Could you check a few things on this model? Use its own coordinates, in mm. Face numbers are marked on the shaded views. A direction names the side the tool comes from. Coordinates: 2 decimals unless noted, no trailing zeros. Order: outer loops, then holes, each group sorted by start corner. A loop starts at its lowest first (then second) coordinate and runs counter-clockwise, first axis right, second up. Notation, with made-up numbers: (54, 27.5) - (78, 27.5) arc R22 ccw to (78, 51.5) - close; hole circle Ø6 at (29, 88). An arc over 180 degrees is marked (long way). One line per item, written item: value. Start each with the question number.
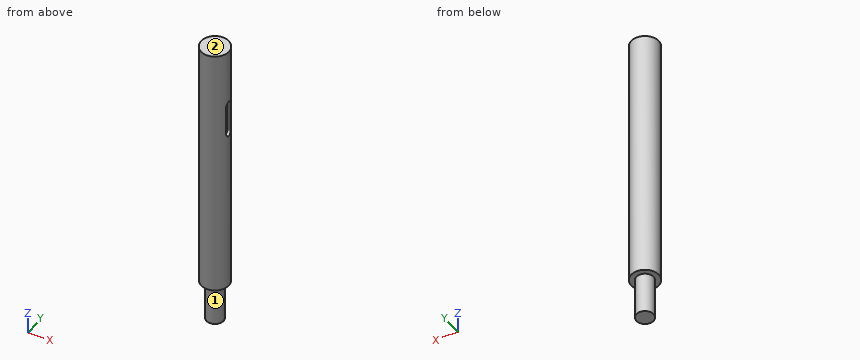
from build123d import *

# Parameters (mm, degrees)
SKETCH_1_R          = 4
EXTRUDE_1_DEPTH     = 75
SKETCH_2_R          = 2.5
EXTRUDE_2_DEPTH     = 12
CUT_EXTRUDE_1_DEPTH = 2


with BuildPart() as part:
    # ｽｹｯﾁ1 → ﾎﾞｽ - 押し出し1 (new body)
    with BuildSketch(Plane.XY):
        Circle(SKETCH_1_R)
    extrude(amount=EXTRUDE_1_DEPTH)

    # ｽｹｯﾁ2 → ﾎﾞｽ - 押し出し2 (add)
    with BuildSketch(Plane(origin=(0, 0, 0), x_dir=(-1, 0, 0), z_dir=(0, 0, -1))):
        Circle(SKETCH_2_R)
    extrude(amount=EXTRUDE_2_DEPTH)

    # ｽｹｯﾁ3 → ｶｯﾄ - 押し出し1 (cut, through all)
    with BuildSketch(Plane(origin=(3, 0, 0), x_dir=(0, 0, -1), z_dir=(1, 0, 0))):
        with BuildLine():
            Line((-57.9, 1.1), (-49.1, 1.1))
            ThreePointArc((-49.1, 1.1), (-48, 0), (-49.1, -1.1))
            Line((-49.1, -1.1), (-57.9, -1.1))
            ThreePointArc((-57.9, -1.1), (-59, 0), (-57.9, 1.1))
        make_face()
    extrude(amount=CUT_EXTRUDE_1_DEPTH, mode=Mode.SUBTRACT)


solid = part.part
Q1. I want a section at B-B on y = 0. Please give me the cut outline in (x, z), then the cut area to 3 significant figures.
Q2. I want a section at A-A on x = 0. Please give me the cut outline in (y, z).
Q3. I'm going to push flat-ended pins straight in: pin 1 (0.9 mm diameter, centred on x = 3, z = 52, fed in from -Y); pin 2 (1.1 mm diameter, centred on y = 0, z = 56, fed in from +X); pin 3 (2 mm diameter, centred on y = 2.5, z = 58.5, fed in from +X). Where does each tip first touch, or does it pass through?
Q4. Which directions (+Z, -Z, +X, -X, +Y, -Y) give clear straight access to the entire face, cutting with the end or side of a thin tool? Please do the marked faces 1 and 2.
Q5. I want a section at C-C on z = 31. Please give me the cut outline in (x, y).
Q6. If I drill on L1, parallel to Z at x = 0, y = 3; L2, parallel to Z at x = 3.5, y = -0.5; L3, parallel to Y at x = 3.5, z = 52, over which ranges is the centre line in solid material (lowest first)?
Values follow:
1. outline: (-4, 0) - (-2.5, 0) - (-2.5, -12) - (2.5, -12) - (2.5, 0) - (4, 0) - (4, 48) - (3, 48) - (3, 59) - (4, 59) - (4, 75) - (-4, 75) - close
1. area: 649 mm^2
2. outline: (-4, 0) - (-2.5, 0) - (-2.5, -12) - (2.5, -12) - (2.5, 0) - (4, 0) - (4, 75) - (-4, 75) - close
3. pin 1: stops at y = -3.08
3. pin 2: stops at x = 3
3. pin 3: stops at x = 3.71
4. face 1: -Z
4. face 2: +Z, +X, -X, +Y, -Y
5. outline: circle Ø8 at (0, 0)
6. L1: z = 0 to 75
6. L2: z = 0 to 48.12, 58.88 to 75
6. L3: y = -1.94 to -1.1, 1.1 to 1.94
